Read the model definition and answer for the solid it produces. Units are mm, in the model's axes. A direction names the side the tool comes from. Coordinates: 2 decimals unless noted, no trailing zeros. Write each loop counter-clockwise with the first axis right and the second up, starting at its lowest first coordinate (ties: lowest second). Pieces come first, ordered by that corner, then holes. Notation, with made-up numbers: (-31.75, 5.5) -> (0.25, 5.5) arc R25 cw to (0.25, 32.5) -> close; hole circle Ø11 at (30, 85.25). An arc over 180 degrees is marked (long way). Use CSV: the item, a comma, the result in double quotes.
Autodesk Inventor part; units mm, degrees
ref_plane "YZ Plane" through (0, 0, 0) normal (1, 0, 0) x (0, 1, 0)
ref_plane "XZ Plane" through (0, 0, 0) normal (0, 1, 0) x (-1, 0, 0)
ref_plane "XY Plane" through (0, 0, 0) normal (0, 0, 1) x (1, 0, 0)
sketch "Sketch1" plane through (0, 0, 0) normal (0, 0, 1) x (1, 0, 0)
  line L0 (-76.6085, 0) -> (76.6085, 0) construction
  line L1 (-48, 0) -> (48, 0)
  line L2 (48, 0) -> (48, 11)
  line L3 (48, 11) -> (-48, 11)
  line L4 (-48, 11) -> (-48, 0)
  point P0 (0, 0)
  point P1 (0, 0)
  point P2 (0, 11)
  dimension "d0" = 96
  dimension "d1" = 11
revolve "Revolution1" add sketch "Sketch1" angle 360 about axis through (-76.6085, 0, 0) along (1, 0, 0)
sketch "Sketch2" plane through (48, 0, 0) normal (1, 0, 0) x (0, 0, -1)
  circle A0 centre (0, 0) radius 22.5
  dimension "d3" = 45
extrude "Extrusion1" add sketch "Sketch2" along normal blind 30
sketch "Sketch3" plane through (0, 0, 0) normal (0, 0, 1) x (1, 0, 0)
  line L0 (78, -22.5) -> (78, 22.5)
  line L1 (78, 27.5) -> (78, -212.5)
  line L2 (48, 22.5) -> (78, 22.5)
  line L3 (48, -22.5) -> (78, -22.5)
  line L4 (78, 27.5) -> (158, 27.5)
  line L5 (158, 27.5) -> (158, -212.5)
  line L6 (78, -212.5) -> (98, -212.5)
  line L7 (158, -212.5) -> (138, -212.5)
  line L8 (118, 27.5) -> (118, -212.5) construction
  line L9 (98, -212.5) -> (98, -362.5)
  line L10 (98, -362.5) -> (138, -362.5)
  line L11 (138, -362.5) -> (138, -212.5)
  line L12 (108, -362.5) -> (128, -362.5)
  line L13 (128, -362.5) -> (128, -492.5)
  line L14 (128, -492.5) -> (108, -492.5)
  line L15 (108, -492.5) -> (108, -362.5)
  line L16 (138, -212.5) -> (98, -212.5)
  point P0 (0, 0)
  point P1 (118, -362.5)
  dimension "d6" = 5
  dimension "d7" = 190
  dimension "d8" = 80
  dimension "d9" = 40
  dimension "d10" = 150
  dimension "d36" = 20
  dimension "d37" = 130
extrude "Extrusion2" add sketch "Sketch3" along normal mid plane 80 contours L0 L1 L4 L5 L7 L16 L6
extrude "Extrusion7" add sketch "Sketch3" along normal mid plane 50 contours L16 L11 L10 L9
extrude "Extrusion8" add sketch "Sketch3" along normal mid plane 20 contours L10 L13 L14 L15
properties part number "simp_burnisher"
1. Each of these flat-tipped pins is pushed along its axis until it touches: pin 1 Ø6 at (y, z) = (-159, -5) entering from -X; pin 2 Ø1.5 at (y, z) = (-258.5, -8) entering from +X; pin 3 Ø1 at (x, y) = (129, -229) entering from +Z. Where does it stop, or does it pass through?
Solutions:
pin 1,"stops at x = 78"
pin 2,"stops at x = 138"
pin 3,"stops at z = 25"
2. A tool of negligible diameter and unlimited length cuts with its end or side. For faces 1 (the flat face through (138, -289, 0)), 2 (the flat face through (118, -427, 10)), 3 (the flat face through (48, 5, -10)), 4 (the flat face through (118, -427, -10)), from which of +Z, -Z, +X, -X, +Y, -Y can it reach the whole face along a straight path? Write none if from no direction.
Solutions:
face 1,"+Z, -Z, +X, -Y"
face 2,"+Z, +X, -X, -Y"
face 3,"-X"
face 4,"-Z, +X, -X, -Y"
3. Find the intervals of material crossed by line 1 along X through (y, z) = (-340, -4.5); line 2 along X through (y, z) = (-421, 2); line 3 along Y through (x, z) = (87, 11.5), in increasing order.
Solutions:
line 1,"x = 98 to 138"
line 2,"x = 108 to 128"
line 3,"y = -212.5 to 27.5"
4. A cutting plane is placed at D-D (y = -206). Give the vertices of the cut face in (x, z), and give its area (3 significant figures).
Solutions:
outline,"(78, -40) -> (158, -40) -> (158, 40) -> (78, 40) -> close"
area,"6,400 mm^2"
5. A cutting plane is placed at C-C (z = -30). Give the vertices of the cut face in (x, y), and give its area (3 significant figures).
Solutions:
outline,"(78, -212.5) -> (158, -212.5) -> (158, 27.5) -> (78, 27.5) -> close"
area,"19,200 mm^2"
6. A cutting plane is placed at A-A (y = 0). Give the vertices of the cut face in (x, z).
Solutions:
outline,"(-48, -11) -> (48, -11) -> (48, -22.5) -> (78, -22.5) -> (78, -40) -> (158, -40) -> (158, 40) -> (78, 40) -> (78, 22.5) -> (48, 22.5) -> (48, 11) -> (-48, 11) -> close"
7. A cutting plane is placed at B-B (z = 0). Give the vertices of the cut face in (x, y).
Solutions:
outline,"(-48, -11) -> (48, -11) -> (48, -22.5) -> (78, -22.5) -> (78, -212.5) -> (98, -212.5) -> (98, -362.5) -> (108, -362.5) -> (108, -492.5) -> (128, -492.5) -> (128, -362.5) -> (138, -362.5) -> (138, -212.5) -> (158, -212.5) -> (158, 27.5) -> (78, 27.5) -> (78, 22.5) -> (48, 22.5) -> (48, 11) -> (-48, 11) -> close"
